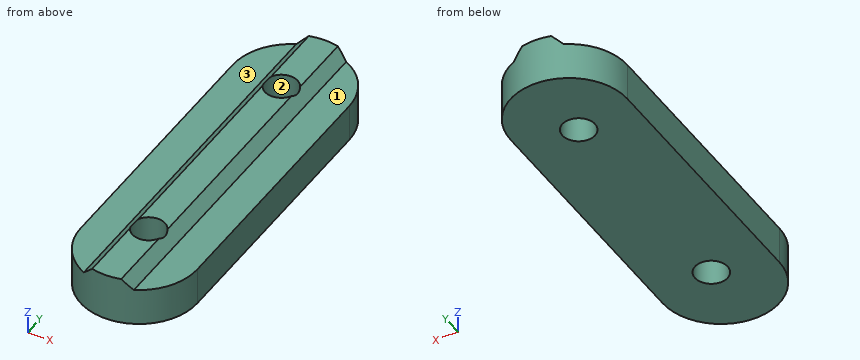
Autodesk Fusion 360 part; units mm, degrees
sketch "Sketch1" plane through (0, 0, 0) normal (0, 0, 1) x (1, 0, 0)
  circle A0 centre (0, -19.85) radius 2.8
  circle A1 centre (0, -10) radius 2.55 construction
  circle A2 centre (0, 0) radius 2.55 construction
  circle A3 centre (0, 10) radius 2.55 construction
  circle A4 centre (0, 19.85) radius 2.8
  circle A5 centre (-10, 0) radius 2.55 construction
  circle A6 centre (-10, 19.85) radius 2.55 construction
  circle A7 centre (-10, -19.85) radius 2.55 construction
  circle A8 centre (10, -19.85) radius 2.55 construction
  circle A9 centre (10, 0) radius 2.55 construction
  circle A10 centre (10, 19.85) radius 2.55 construction
  circle A11 centre (-20, -19.85) radius 3.6
  circle A12 centre (-20, 19.85) radius 2.55
  circle A13 centre (20, 19.85) radius 2.55
  circle A14 centre (20, -19.85) radius 3.6
  line L0 (-32.75, 29.75) -> (-32.75, -29.75)
  arc A15 (-32.75, -29.75) -> (-29.75, -32.75) centre (-29.75, -29.75) ccw
  line L1 (0, -32.75) -> (0, -32.75)
  arc A16 (-29.75, 32.75) -> (-32.75, 29.75) centre (-29.75, 29.75) ccw
  line L2 (0, 32.75) -> (0, 32.75)
  arc A17 (32.75, 29.75) -> (29.75, 32.75) centre (29.75, 29.75) ccw
  line L3 (32.75, -29.75) -> (32.75, 29.75)
  arc A18 (29.75, -32.75) -> (32.75, -29.75) centre (29.75, -29.75) ccw
  line L4 (26.2, -23.4) -> (26.2, -16.9)
  line L5 (29.2, -16.9) -> (29.2, -23.4)
  line L6 (29.2, 3.25) -> (29.2, -3.25)
  line L7 (26.2, -3.25) -> (26.2, 3.25)
  line L8 (26.2, 16.9) -> (26.2, 23.4)
  line L9 (29.2, 23.4) -> (29.2, 16.9)
  arc A19 (29.2, 23.4) -> (26.2, 23.4) centre (27.7, 23.4) ccw
  arc A20 (26.2, 16.9) -> (29.2, 16.9) centre (27.7, 16.9) ccw
  arc A21 (29.2, 3.25) -> (26.2, 3.25) centre (27.7, 3.25) ccw
  arc A22 (26.2, -3.25) -> (29.2, -3.25) centre (27.7, -3.25) ccw
  arc A23 (29.2, -16.9) -> (26.2, -16.9) centre (27.7, -16.9) ccw
  arc A24 (26.2, -23.4) -> (29.2, -23.4) centre (27.7, -23.4) ccw
  arc A25 (17.5, -10.32) -> (22.5, -10.32) centre (20, -10.32) ccw
  arc A26 (22.5, 10.32) -> (17.5, 10.32) centre (20, 10.32) ccw
  line L10 (17.5, -10.32) -> (17.5, 10.32)
  line L11 (22.5, 10.32) -> (22.5, -10.32)
  arc A27 (-17.5, 10.32) -> (-22.5, 10.32) centre (-20, 10.32) ccw
  arc A28 (-22.5, -10.32) -> (-17.5, -10.32) centre (-20, -10.32) ccw
  line L12 (-17.5, 10.32) -> (-17.5, -10.32)
  line L13 (-22.5, -10.32) -> (-22.5, 10.32)
  arc A29 (-26.2, 3.25) -> (-29.2, 3.25) centre (-27.7, 3.25) ccw
  arc A30 (-29.2, -3.25) -> (-26.2, -3.25) centre (-27.7, -3.25) ccw
  line L14 (-29.2, -3.25) -> (-29.2, 3.25)
  line L15 (-26.2, 3.25) -> (-26.2, -3.25)
  arc A31 (-26.2, -16.9) -> (-29.2, -16.9) centre (-27.7, -16.9) ccw
  arc A32 (-29.2, -23.4) -> (-26.2, -23.4) centre (-27.7, -23.4) ccw
  line L16 (-26.2, -16.9) -> (-26.2, -23.4)
  line L17 (-29.2, -23.4) -> (-29.2, -16.9)
  arc A33 (-29.2, 16.9) -> (-26.2, 16.9) centre (-27.7, 16.9) ccw
  arc A34 (-26.2, 23.4) -> (-29.2, 23.4) centre (-27.7, 23.4) ccw
  line L18 (-29.2, 16.9) -> (-29.2, 23.4)
  line L19 (-26.2, 23.4) -> (-26.2, 16.9)
  line L20 (0, 32.75) -> (0, -32.75) construction
  line L21 (-10, 32.75) -> (-10, -32.75)
  line L22 (10, 32.75) -> (10, -32.75)
  arc A35 (-9.9939, -22.4) -> (9.9939, -22.4) centre (0, -22.75) ccw
  arc A36 (9.9939, 22.4) -> (-9.9939, 22.4) centre (0, 22.75) ccw
  line L23 (-29.75, -32.75) -> (29.75, -32.75)
  line L24 (-29.75, 32.75) -> (29.75, 32.75)
  dimension "d3" = 5.6
  dimension "d4" = 5.6
sketch "Sketch2" plane through (0, 0, 0) normal (0, 1, 0) x (1, 0, 0)
  line L0 (4.2864, -6.4) -> (-4.2864, -6.4)
  line L1 (4.2864, -6.4) -> (2.4864, -8.2)
  line L2 (2.4864, -24.6) -> (-2.4864, -24.6)
  line L3 (-2.4864, -8.2) -> (-4.2864, -6.4)
  circle A0 centre (0, -16.4) radius 2.1 construction
  line L4 (2.4864, -8.2) -> (-2.4864, -8.2)
  line L5 (4.2864, -26.4) -> (2.4864, -24.6)
  line L6 (4.2864, -26.4) -> (-4.2864, -26.4)
  line L7 (-2.4864, -24.6) -> (-4.2864, -26.4)
  line L8 (3.9, -19.24) -> (3.9, -13.56) construction
  line L9 (-6.56, -21.9) -> (-8.2, -21.9) construction
  line L10 (8.2, -19.24) -> (8.2, -21.9) construction
  line L11 (-3.9, -13.56) -> (-3.9, -19.24) construction
  line L12 (8.2, -21.9) -> (6.56, -21.9) construction
  line L13 (-5.5, -24.6) -> (-5.5, -22.96) construction
  line L14 (2.84, -12.5) -> (-2.84, -12.5) construction
  line L15 (10, -26.4) -> (10, -21.04) construction
  line L16 (6.56, -10.9) -> (8.2, -10.9) construction
  line L17 (6.56, -21.9) -> (3.9, -19.24) construction
  line L18 (5.5, -24.6) -> (2.84, -24.6) construction
  line L19 (-2.84, -12.5) -> (-5.5, -9.84) construction
  line L20 (-2.84, -24.6) -> (-5.5, -24.6) construction
  line L21 (-3.9, -19.24) -> (-6.56, -21.9) construction
  line L22 (-6.56, -10.9) -> (-3.9, -13.56) construction
  line L23 (-5.5, -22.96) -> (-2.84, -20.3) construction
  line L24 (-10, -26.4) -> (-4.64, -26.4) construction
  line L25 (-5.5, -8.2) -> (-2.84, -8.2) construction
  line L26 (-4.64, -6.4) -> (-10, -6.4) construction
  line L27 (-8.2, -13.56) -> (-8.2, -10.9) construction
  line L28 (5.5, -9.84) -> (2.84, -12.5) construction
  line L29 (-8.2, -10.9) -> (-6.56, -10.9) construction
  line L30 (-10, -6.4) -> (-10, -11.76) construction
  line L31 (5.5, -8.2) -> (5.5, -9.84) construction
  line L32 (-10, -11.76) -> (-8.2, -13.56) construction
  line L33 (10, -21.04) -> (8.2, -19.24) construction
  line L34 (-2.84, -20.3) -> (2.84, -20.3) construction
  line L35 (-8.2, -19.24) -> (-10, -21.04) construction
  line L36 (-8.2, -21.9) -> (-8.2, -19.24) construction
  line L37 (2.84, -8.2) -> (5.5, -8.2) construction
  line L38 (-10, -21.04) -> (-10, -26.4) construction
  line L39 (8.2, -10.9) -> (8.2, -13.56) construction
  line L40 (2.84, -24.6) -> (4.64, -26.4) construction
  line L41 (-5.5, -9.84) -> (-5.5, -8.2) construction
  line L42 (3.9, -13.56) -> (6.56, -10.9) construction
  line L43 (4.64, -26.4) -> (10, -26.4) construction
  line L44 (10, -6.4) -> (4.64, -6.4) construction
  line L45 (5.5, -22.96) -> (5.5, -24.6) construction
  line L46 (2.84, -20.3) -> (5.5, -22.96) construction
  line L47 (-4.64, -26.4) -> (-2.84, -24.6) construction
  line L48 (10, -11.76) -> (10, -6.4) construction
  line L49 (-2.84, -8.2) -> (-4.64, -6.4) construction
  line L50 (8.2, -13.56) -> (10, -11.76) construction
  line L51 (4.64, -6.4) -> (2.84, -8.2) construction
extrude "Extrude1" add sketch "Sketch1" along normal blind 6.4 contours L21 L22 A35 A36
extrude "Extrude2" add sketch "Sketch2" along normal mid plane 65.5 contours L0 L1 L3 L4
extrude "Extrude3" cut sketch "Sketch1" along normal through all contours A0 | A4
extrude "Extrude4" cut sketch "Sketch1" along normal through all contours L21 A36 L24 | L21 A35 L23 | L22 A36 L24 | L22 A35 L23
Check sheet for the modelled part. Datum: model origin and axes. Units: mm. Face numbers are marked on the shaded views. A direction names the side the tool comes from. Give positions to 0.01 mm unless a question says otherwise; leave off trailing zeros. Loops run counter-clockwise (first coordinate to the right, second up) from the corner with the lowest first, then second, coordinate; pieces in that order, holes last. Notation, with made-up numbers: (1.5, 5.25) - (56.5, 5.25) arc R21 ccw to (56.5, 26.25) - close; hole circle Ø9 at (-6, -17.75). An arc over 180 degrees is marked (long way). One line per question, with ' | ' between items. Start each with the question number.
1. Cross-section at D-D, the plane y = -11. Enter the section's corners in (x, z).
2. Gauge pin test, flat ends, axial feed: pin 1 Ø3 at (x, y) = (5.5, 4.5) entering from +Z; pin 2 Ø4.5 at (x, y) = (-6, 4.5) entering from +Z; pin 3 Ø1.5 at (x, z) = (-3, 2.5) entering from -Y; pin 4 Ø4.5 at (x, y) = (0, -19.85) entering from -Z. Record the tip position at first contact, or that the pin passes through.
3. Cross-section at A-A, the plane x = 0. Enter the section's corners in (y, z).
4. Cross-section at C-C, the plane z = 3.75. Enter the section's corners in (x, y), plus the area to 3 significant figures.
5. Cross-section at B-B, the plane y = -18. Enter the section's corners in (x, z), plus the area to 3 significant figures.
6. Material ranges on line 1 along Y through (x, z) = (0, 6.5); line 2 along X through (y, z) = (-19.85, 4.5); line 3 along Y through (x, z) = (1.75, 2), recorded low to high. Write a range as [from, to].
7. Set-up check for the marked faces 1, 2 and 3: record each of +Z, -Z, +X, -X, +Y, -Y from which the full face is reachable in a straight line by a thin tool's end or side.
Check result:
1) outline: (-10, 0) - (10, 0) - (10, 6.4) - (4.29, 6.4) - (2.49, 8.2) - (-2.49, 8.2) - (-4.29, 6.4) - (-10, 6.4) - close
2) pin 1: stops at z = 6.69 | pin 2: stops at z = 6.94 | pin 3: stops at y = -32.49 | pin 4: passes through
3) outline: (-32.75, 0) - (-22.65, 0) - (-22.65, 8.2) - (-32.75, 8.2) - close; (-17.05, 0) - (17.05, 0) - (17.05, 8.2) - (-17.05, 8.2) - close; (22.65, 0) - (32.75, 0) - (32.75, 8.2) - (22.65, 8.2) - close
4) outline: (-10, -22.75) arc R10 ccw to (10, -22.75) - (10, 22.75) arc R10 ccw to (-10, 22.75) - close; hole circle Ø5.6 at (0, -19.85); hole circle Ø5.6 at (0, 19.85) | area: 1,170 mm2
5) outline: (-10, 0) - (-2.1, 0) - (-2.1, 8.2) - (-2.49, 8.2) - (-4.29, 6.4) - (-10, 6.4) - close; (2.1, 0) - (10, 0) - (10, 6.4) - (4.29, 6.4) - (2.49, 8.2) - (2.1, 8.2) - close | area: 106 mm2
6) line 1: y = [-32.75, -22.65], [-17.05, 17.05], [22.65, 32.75] | line 2: x = [-10, -2.8], [2.8, 10] | line 3: y = [-32.6, -22.04], [-17.66, 17.66], [22.04, 32.6]
7) face 1: +Z, +X, +Y, -Y | face 2: +Z, -Z | face 3: +Z, -X, +Y, -Y
